Model file for the job. Use its own axes, mm. A direction names the side the tool comes from. Coordinates: 2 decimals unless noted, no trailing zeros. Answer as a JSON object with one key per item and string values. Group by question number.
from build123d import *

# Parameters (mm, degrees)
BOSS_EXTRUDE1_DEPTH = 110
BOSS_EXTRUDE2_DEPTH = 3
LPATTERN2_COUNT     = 17
LPATTERN2_PITCH     = 6


with BuildPart() as part:
    # Sketch2 → Boss-Extrude1 (new body)
    with BuildSketch(Plane(origin=(0, 0, 0), x_dir=(1, 0, 0), z_dir=(0, 1, 0))):
        with BuildLine():
            Line((25, 0), (37, 0))
            Line((37, 0), (37, 55))
            ThreePointArc((37, 55), (34.071067812, 62.071067812), (27, 65))
            Line((27, 65), (-27, 65))
            ThreePointArc((-27, 65), (-34.071067812, 62.071067812), (-37, 55))
            Line((-37, 55), (-37, 0))
            Line((-37, 0), (-25, 0))
            ThreePointArc((-25, 0), (0, 25), (25, 0))
        make_face()
    extrude(amount=BOSS_EXTRUDE1_DEPTH)

    # Sketch3 → Boss-Extrude2 (add)
    with BuildSketch(Plane.XZ):
        with BuildLine():
            Line((-41, 0), (-41, -55))
            ThreePointArc((-41, -55), (-36.899494937, -64.899494937), (-27, -69))
            Line((-27, -69), (27, -69))
            ThreePointArc((27, -69), (36.899494937, -64.899494937), (41, -55))
            Line((41, -55), (41, 0))
            Line((41, 0), (37, 0))
            Line((37, 0), (37, -55))
            ThreePointArc((37, -55), (34.071067812, -62.071067812), (27, -65))
            Line((27, -65), (-27, -65))
            ThreePointArc((-27, -65), (-34.071067812, -62.071067812), (-37, -55))
            Line((-37, -55), (-37, 0))
            Line((-37, 0), (-41, 0))
        make_face()
    boss_extrude2 = extrude(amount=-BOSS_EXTRUDE2_DEPTH)

    # LPattern2: Boss-Extrude2 ×17
    with Locations(*[(0, i * LPATTERN2_PITCH, 0) for i in range(1, LPATTERN2_COUNT)]):
        add(boss_extrude2)


solid = part.part
(1) Pin check, flat tips, straight feed: pin 1 (3.5 mm diameter, centred on x = 3, y = 46, fed in from -Z); pin 2 (1.5 mm diameter, centred on y = 47, z = -29.5, fed in from -X); pin 3 (1.5 mm diameter, centred on x = 4.5, y = 4, fed in from -Z); pin 4 (2 mm diameter, centred on x = 11, y = 77.5, fed in from +Z). Stop position of each tip, or through.
(2) Wall check: probe 1 along X at (y, z) = (16.5, -3); probe 2 along X at (y, z) = (47, -19.5); probe 3 along X at (y, z) = (11, -47.5). Give the ranges that are in metal, low to high.
(3) 3-axis set-ups, long thin cutter, end or side, ignore diameter. For faces 3 (the face through (-37, 4, -28)), 4 (the face through (36.8, 37.5, -65)), 5 (the face through (-33.99, 4.48, -62.15)), 6 (the face through (0, 10, -65)), 7 (the face through (34.15, 58.48, -61.99)): which of +Z, -Z, +X, -X, +Y, -Y reach the whole face in a straight line?
(4) Pull direction Y, two halves, no side cores. Call faces 1 (the face through (-33.99, 34.48, -62.15)), 2 (the face through (0, 79, -69)): released by +Y, released by -Y, zero draft, split by the parting line, or undercut.
Results found:
{
 "1": {"pin 1": "stops at z = -69", "pin 2": "stops at x = -37", "pin 3": "stops at z = -65", "pin 4": "stops at z = -21.93"},
 "2": {"probe 1": "x = -37 to -24.82, 24.82 to 37", "probe 2": "x = -37 to -15.64, 15.64 to 37", "probe 3": "x = -37 to 37"},
 "3": {"face 3": "+Z, -Z, -X", "face 4": "-Z, +X, +Y, -Y", "face 5": "-Z, -X", "face 6": "-Z, +X, -X", "face 7": "-Z, +X"},
 "4": {"face 1": "undercut", "face 2": "zero draft"}
}
